The model under review builds one solid part; all positions refer to its coordinate system, in mm. A direction names the side the tool comes from. Round coordinates to 2 decimals unless told otherwise and drop trailing zeros. Loops run counter-clockwise (first coordinate to the right, second up) from the corner with the lowest first, then second, coordinate; pieces in that order, holes last. Notation, with made-up numbers: (89, 16) -> (119, 16) arc R15 ccw to (119, 38) -> close; hole circle Ø2 at (39.5, -39.75). An arc over 180 degrees is marked (long way). Write each question's results on one line, items separated by ' | '. Start each with the question number.
Item 1: Tool access review of faces 1 (the flat face through (0, 1, 24)), 2 (the flat face through (0, 1, 21)): name each direction out of +Z, -Z, +X, -X, +Y, -Y from which nothing blocks a thin tool from reaching the whole face with its end or side.
Item 2: We need section B-B (x = -1.25). Give the boundary of the cut face in (y, z), and give its area (3 significant figures).
Item 3: For L1, parallel to Z at x = 1.5, y = 1.8; L2, parallel to X at y = 2.2, z = -1.5; L3, parallel to X at y = 0.25, z = -20, list the stretches that pass through material, from the lowest coordinate up. Write a range as from..to.
Item 4: Clearance check with a flat-ended pin moving along its axis: pin 1 Ø6 at (x, z) = (-4.5, -11.5) entering from +Y. State where the tip first meets the part, or that it passes through.
Item 5: Mouldability with a two-part tool opening along X and no side actions: class faces 3 (the cylindrical face through (11.05, 1.52, 23.57)), 4 (the cylindrical face through (-11.05, 1.52, -23.57)), 5 (the flat face through (0, 1, -21)) as pulls with the +X half, pulls with the -X half, needs draft (parallel to the pull), parting line crosses it, or undercut.
Item 6: We need section A-A (z = 6). Give the boundary of the cut face in (x, y), and give its area (3 significant figures).
Item 7: We need section C-C (y = 2.15). Give the boundary of the cut face in (x, z), and give its area (3 significant figures).
Autodesk Inventor part; units mm, degrees
ref_plane "YZ Plane" through (0, 0, 0) normal (1, 0, 0) x (0, 1, 0)
ref_plane "XZ Plane" through (0, 0, 0) normal (0, 1, 0) x (-1, 0, 0)
ref_plane "XY Plane" through (0, 0, 0) normal (0, 0, 1) x (1, 0, 0)
sketch "Sketch1" plane through (0, 0, 0) normal (0, 1, 0) x (-1, 0, 0)
  line L0 (11.5, 24) -> (-11.5, 24)
  line L1 (-11.5, 24) -> (-11.5, -24)
  line L2 (-11.5, -24) -> (11.5, -24)
  line L3 (11.5, -24) -> (11.5, 24)
  line L4 (11.5, 24) -> (-11.5, -24) construction
  line L5 (-11.5, 24) -> (11.5, -24) construction
  line L6 (-8.5, 21) -> (8.5, 21)
  line L7 (8.5, 21) -> (8.5, -21)
  line L8 (8.5, -21) -> (-8.5, -21)
  line L9 (-8.5, -21) -> (-8.5, 21)
  line L10 (-8.5, 21) -> (8.5, -21) construction
  line L11 (8.5, 21) -> (-8.5, -21) construction
  line L12 (0, 0) -> (-8.5, 0) construction
  circle A0 centre (0, -12) radius 1.5
  circle A1 centre (0, 12) radius 1.5
  line L13 (17.5, 30) -> (-17.5, 30)
  line L14 (-17.5, 30) -> (-17.5, -30)
  line L15 (-17.5, -30) -> (17.5, -30)
  line L16 (17.5, -30) -> (17.5, 30)
  line L17 (17.5, 30) -> (-17.5, -30) construction
  line L18 (-17.5, 30) -> (17.5, -30) construction
  circle A2 centre (14.5, 27) radius 1.5
  circle A3 centre (-14.5, 27) radius 1.5
  circle A4 centre (14.5, -27) radius 1.5
  circle A5 centre (-14.5, -27) radius 1.5
  dimension "d0" = 23
  dimension "d1" = 48
  dimension "d3" = 3
  dimension "d4" = 3
  dimension "d5" = 3
  dimension "d6" = 12
  dimension "d9" = 6
  dimension "d10" = 6
  dimension "d13" = 3
  dimension "d14" = 3
  dimension "d15" = 3
  dimension "d16" = 3
  dimension "d17" = 3
  dimension "d18" = 3
extrude "Extrusion1" add sketch "Sketch1" along normal blind 3 contours L3 L2 L1 L0
fillet "Fillet2" radius 1.5 4 edges at (11.5, 1.5, 24) (-11.5, 1.5, 24) (-11.5, 1.5, -24) (11.5, 1.5, -24)
fillet "Fillet3" radius 1.5 4 edges at (8.5, 1.5, -21) (8.5, 1.5, 21) (-8.5, 1.5, 21) (-8.5, 1.5, -21)
properties part number "Chamber"
Here are the results:
1) face 1: +Z, +X, -X, +Y, -Y | face 2: +Y, -Y
2) outline: (0, -24) -> (3, -24) -> (3, -21) -> (0, -21) -> close; (0, 21) -> (3, 21) -> (3, 24) -> (0, 24) -> close | area: 18.0 mm2
3) L1: z = -24..-21, 21..24 | L2: x = -11.5..-8.5, 8.5..11.5 | L3: x = -11.5..-8.41, 8.41..11.5
4) pin 1: passes through
5) face 3: pulls with the +X half | face 4: pulls with the -X half | face 5: undercut
6) outline: (-11.5, 0) -> (-8.5, 0) -> (-8.5, 3) -> (-11.5, 3) -> close; (8.5, 0) -> (11.5, 0) -> (11.5, 3) -> (8.5, 3) -> close | area: 18.0 mm2
7) outline: (-11.5, -22.5) arc R1.5 ccw to (-10, -24) -> (10, -24) arc R1.5 ccw to (11.5, -22.5) -> (11.5, 22.5) arc R1.5 ccw to (10, 24) -> (-10, 24) arc R1.5 ccw to (-11.5, 22.5) -> close; hole (-8.5, -19.5) arc R1.5 ccw to (-7, -21) -> (7, -21) arc R1.5 ccw to (8.5, -19.5) -> (8.5, 19.5) arc R1.5 ccw to (7, 21) -> (-7, 21) arc R1.5 ccw to (-8.5, 19.5) -> close | area: 390 mm2
